Could you check a few things on this model? Use its own coordinates, in mm. A direction names the side the tool comes from. Give positions to 0.01 mm unless a question says otherwise; leave off trailing zeros. Write each loop counter-clockwise with the first axis right and the second up, starting at its lowest first coordinate (ties: lowest second). Pieces come first, ordered by that corner, then holes. Notation, with made-up numbers: (47.25, 36.5) - (101.25, 36.5) arc R27 cw to (101.25, 75.5) - close; hole circle Ø9 at (29.5, 28.25). An arc over 180 degrees is marked (long way). Answer in a Markdown table with one row per item.
from build123d import *

# Parameters (mm, degrees)
BOSS_EXTRUDE1_DEPTH     = 5
CUT_EXTRUDE1_DEPTH      = 48.542086618
SKETCH3_R               = 2
CUT_EXTRUDE2_DEPTH      = 48.542086618
FILLET1_R               = 2
SKETCH5_W               = 12
SKETCH5_H               = 7
BOSS_EXTRUDE2_DEPTH     = 15
CUT_EXTRUDE3_DEPTH      = 61.835844697
CUT_EXTRUDE3_DEPTH_BACK = 61.835844697
SKETCH4_R               = 1.6
FILLET2_R               = 5


with BuildPart() as part:
    # Sketch1 → Boss-Extrude1 (new, symmetric)
    with BuildSketch(Plane(origin=(0, 0, 0), x_dir=(0, 0, -1), z_dir=(1, 0, 0))):
        with BuildLine():
            Line((22, -13.5), (30, -13.5))
            Line((30, -13.5), (30, -16.5))
            Line((30, -16.5), (-30, -16.5))
            Line((-30, -16.5), (-30, -13.5))
            Line((-30, -13.5), (-22, -13.5))
            Line((-22, -13.5), (-22, 13.5))
            ThreePointArc((-22, 13.5), (0, 35.5), (22, 13.5))
            Line((22, 13.5), (22, -13.5))
        make_face()
    extrude(amount=BOSS_EXTRUDE1_DEPTH, both=True)

    # Sketch2 → Cut-Extrude1 (cut, through all)
    with BuildSketch(Plane(origin=(5, 0, 0), x_dir=(0, 0, -1), z_dir=(1, 0, 0))):
        with BuildLine():
            Line((-8.139410298, 1.5), (-8.139410298, -9.5))
            Line((-8.139410298, -9.5), (8.139410298, -9.5))
            Line((8.139410298, -9.5), (8.139410298, 1.5))
            ThreePointArc((8.139410298, 1.5), (0, 28), (-8.139410298, 1.5))
        make_face()
    extrude(amount=-CUT_EXTRUDE1_DEPTH, mode=Mode.SUBTRACT)

    # Sketch3 → Cut-Extrude2 (cut, through all)
    with BuildSketch(Plane.ZY.offset(5)):
        with Locations((17.5, 13.5)):
            Circle(SKETCH3_R)
        with Locations((-17.5, 13.5)):
            Circle(SKETCH3_R)
    extrude(amount=-CUT_EXTRUDE2_DEPTH, mode=Mode.SUBTRACT)

    # Fillet1
    fillet1_edges = [part.edges().sort_by_distance(p)[0] for p in [
        (0, -13.5, -22),
        (0, -13.5, 22),
    ]]
    fillet(fillet1_edges, radius=FILLET1_R)

    # Sketch5 → Boss-Extrude2 (add)
    with BuildSketch(Plane(origin=(5, 0, 0), x_dir=(0, 0, -1), z_dir=(1, 0, 0))):
        with Locations((0, -13)):
            Rectangle(SKETCH5_W, SKETCH5_H)
    extrude(amount=BOSS_EXTRUDE2_DEPTH)

    # Sketch4 → Cut-Extrude3 (cut, two sides: drawn at the far end of the back side and taken through both)
    with BuildSketch(Plane(origin=(0, -13.5, 0), x_dir=(1, 0, 0), z_dir=(0, 1, 0)).offset(-CUT_EXTRUDE3_DEPTH_BACK)):
        with Locations(Location((0, 26.8, 0), (0, 0, 270))):
            Circle(SKETCH4_R)
        with Locations(Location((0, -26.8, 0), (0, 0, 270))):
            Circle(SKETCH4_R)
        with Locations(Location((15.988182788, 0, 0), (0, 0, 270))):
            Circle(SKETCH4_R)
    extrude(amount=CUT_EXTRUDE3_DEPTH + CUT_EXTRUDE3_DEPTH_BACK, mode=Mode.SUBTRACT)

    # Fillet2
    fillet2_edges = [part.edges().sort_by_distance(p)[0] for p in [
        (5, -13, -6),
        (5, -13, 6),
    ]]
    fillet(fillet2_edges, radius=FILLET2_R)


solid = part.part
1) On a 3-axis mill with a long thin cutter (end or side, diameter ignored), from which of +Z, -Z, +X, -X, +Y, -Y can I reach the whole of each face in a straight line? I mean faces 1 (the face through (15, -13, -6)), 2 (the face through (0, 1, -22)), 3 (the face through (5, 4, -14)), 4 (the face through (1.2, -13.5, 28.4)), 5 (the face through (1, -4, -8.139)). Say none if no direction works.
Check values:
| item | result |
|---|---|
| face 1 | -Z, +X, +Y, -Y |
| face 2 | -Z, +X, -X, +Y |
| face 3 | +X, +Y |
| face 4 | +Z, +X, -X, +Y |
| face 5 | +X, -X |
2) Imagine slicing it at B-B (y = -8). List the corners of the cut face in (x, z) for me.
Check values:
| item | result |
|---|---|
| outline | (-5, -22) - (5, -22) - (5, -11) arc R5 cw to (5.9, -8.14) - (-5, -8.14) - close; (-5, 8.14) - (5.9, 8.14) arc R5 cw to (5, 11) - (5, 22) - (-5, 22) - close |
3) If I drill on line 1 (Z direction, x = 0, y = -15.85); line 2 (Y direction, x = 2.25, z = 0); line 3 (X direction, y = -11.25, z = 0), over which ranges is the centre line in solid material (lowest first)?
Check values:
| item | result |
|---|---|
| line 1 | z = -30 to -28.4, -25.2 to 25.2, 28.4 to 30 |
| line 2 | y = -16.5 to -9.5, 28 to 35.5 |
| line 3 | x = -5 to 14.39, 17.59 to 20 |
4) Will these pins go through, and if not, where does the flat tip stop? P1, Ø5.5, axis at x = 14.5, y = -11.5, coming from the -Z side; P2, Ø3.5, axis at y = 13.5, z = 17.5, coming from the +X side; P3, Ø1.8, axis at x = -1.5, z = 26, coming from the +Y side; P4, Ø8, axis at x = -1.5, y = 7, coming from the -Z side.
Check values:
| item | result |
|---|---|
| P1 | stops at z = -6 |
| P2 | passes through |
| P3 | stops at y = -13.5 |
| P4 | stops at z = -22 |
5) Imagine slicing it at C-C (x = 2.75). List the corners of the cut face in (y, z) for me.
Check values:
| item | result |
|---|---|
| outline | (-16.5, -30) - (-13.5, -30) - (-13.5, -24) arc R2 cw to (-11.5, -22) - (13.5, -22) arc R22 ccw to (13.5, 22) - (-11.5, 22) arc R2 cw to (-13.5, 24) - (-13.5, 30) - (-16.5, 30) - close; hole (-9.5, -8.14) - (1.5, -8.14) arc R14.5 ccw (long way) to (1.5, 8.14) - (-9.5, 8.14) - close; hole circle Ø4 at (13.5, -17.5); hole circle Ø4 at (13.5, 17.5) |
6) Imagine slicing it at D-D (z = 0). List the corners of the cut face in (x, y) for me.
Check values:
| item | result |
|---|---|
| outline | (-5, -16.5) - (14.39, -16.5) - (14.39, -9.5) - (-5, -9.5) - close; (-5, 28) - (5, 28) - (5, 35.5) - (-5, 35.5) - close; (17.59, -16.5) - (20, -16.5) - (20, -9.5) - (17.59, -9.5) - close |
7) Imagine slicing it at A-A (z = -26.8). List the corners of the cut face in (x, y) for me.
Check values:
| item | result |
|---|---|
| outline | (-5, -16.5) - (-1.6, -16.5) - (-1.6, -13.5) - (-5, -13.5) - close; (1.6, -16.5) - (5, -16.5) - (5, -13.5) - (1.6, -13.5) - close |
8) We'd pull the mould along Y, two halves only. Please class faces 6 (the face through (0.07, 35.495, 0.484)), 7 (the face through (15, -13, 6)), 8 (the face through (8, -9.5, 0)): +Y half, -Y half, draft (parallel to the pull), parting line (faces both ways), or undercut.
Check values:
| item | result |
|---|---|
| face 6 | +Y half |
| face 7 | draft |
| face 8 | undercut |
